from build123d import *

# Parameters (mm, degrees)
F0_W      = 36.8749946356
F0_H      = 46.3530421257
F1_DEPTH  = 43.4907004237
F4_DEPTH  = 25.4
F4_FACE_W = 50.4002720118
F4_FACE_H = 95.7473944873
F6_DEPTH  = 80.4695729166


with BuildPart() as f1:
    # F0 (on Top) → F1 (new body)
    with BuildSketch(Plane.XY):
        with Locations((18.4374973178, -11.0187307)):
            Rectangle(F0_W, F0_H)
    extrude(amount=F1_DEPTH)


with BuildPart() as f4:
    # F3 (on Front) → F4 (new body)
    with BuildSketch(Plane.XZ):
        Polygon((-21.5003099293, 85.1215198636), (-21.5003099293, 46.1357757449), (-21.5003099293, -10.6258746237), (28.8999620825, -10.6258746237), (28.8999620825, 85.1215198636), align=None)
    extrude(amount=F4_DEPTH)

    # F4_face (on face) + F5 (on Front) → F6 (cut)
    with BuildSketch(Plane(origin=(3.6998260766, -25.4, 37.24782262), x_dir=(1, 0, 0), z_dir=(0, -1, 0))):
        Rectangle(F4_FACE_W, F4_FACE_H)
    with BuildSketch(Plane.XZ):
        Polygon((-4.3523218483, 0), (-4.3523218483, -10.5397570878), (12.7652771771, -10.5397570878), (12.7652771771, 34.8452031612), (-4.3523218483, 34.8452031612), align=None)
    extrude(amount=F6_DEPTH, mode=Mode.SUBTRACT)


solid = f4.part
The listing builds one solid part. Answer for the finished solid, in the listing's coordinates (mm). A direction names the side the tool comes from. Coordinates: 2 decimals unless noted, no trailing zeros. Loops run counter-clockwise (first coordinate to the right, second up) from the corner with the lowest first, then second, coordinate; pieces in that order, holes last.
1) Find the intervals of material crossed by L1, parallel to X at y = -16, z = 7, in increasing order.
2) Find section B-B on x = 2.5. Write down the section's boundary in (y, z).
3) Find section A-A on y = -20.5. Write down the section's boundary in (x, z).
4) Determine the mould class of faces 1 (the face through (4, -13, 34.845)), 2 (the face through (4, -13, 85.122)), 3 (the face through (-21.5, -13, 38)) for opening direction Z: pulls with the +Z half, pulls with the -Z half, needs draft (parallel to the pull), parting line crosses it, or undercut.
5) Find section C-C on z = 29. Write down the section's boundary in (x, y), then the cut area to 3 significant figures.
6) A tool of negligible diameter and unlimited length cuts with its end or side. For faces 4 (the face through (3, 0, 38)), 5 (the face through (-4.352, -13, 12)), from which of +Z, -Z, +X, -X, +Y, -Y can it reach the whole face along a straight path? Write none if from no direction.
Values:
1. L1: x = -21.5 to -4.35, 12.77 to 28.9
2. outline: (-25.4, -10.63) - (0, -10.63) - (0, -10.54) - (-25.4, -10.54) - close; (-25.4, 34.85) - (0, 34.85) - (0, 85.12) - (-25.4, 85.12) - close
3. outline: (-21.5, -10.63) - (28.9, -10.63) - (28.9, 85.12) - (-21.5, 85.12) - close; hole (-4.35, -10.54) - (12.77, -10.54) - (12.77, 34.85) - (-4.35, 34.85) - close
4. face 1: undercut
4. face 2: pulls with the +Z half
4. face 3: needs draft
5. outline: (-21.5, -25.4) - (-4.35, -25.4) - (-4.35, 0) - (-21.5, 0) - close; (12.77, -25.4) - (28.9, -25.4) - (28.9, 0) - (12.77, 0) - close
5. area: 845 mm2
6. face 4: +Z, -Z, +X, -X, +Y
6. face 5: +Y, -Y
